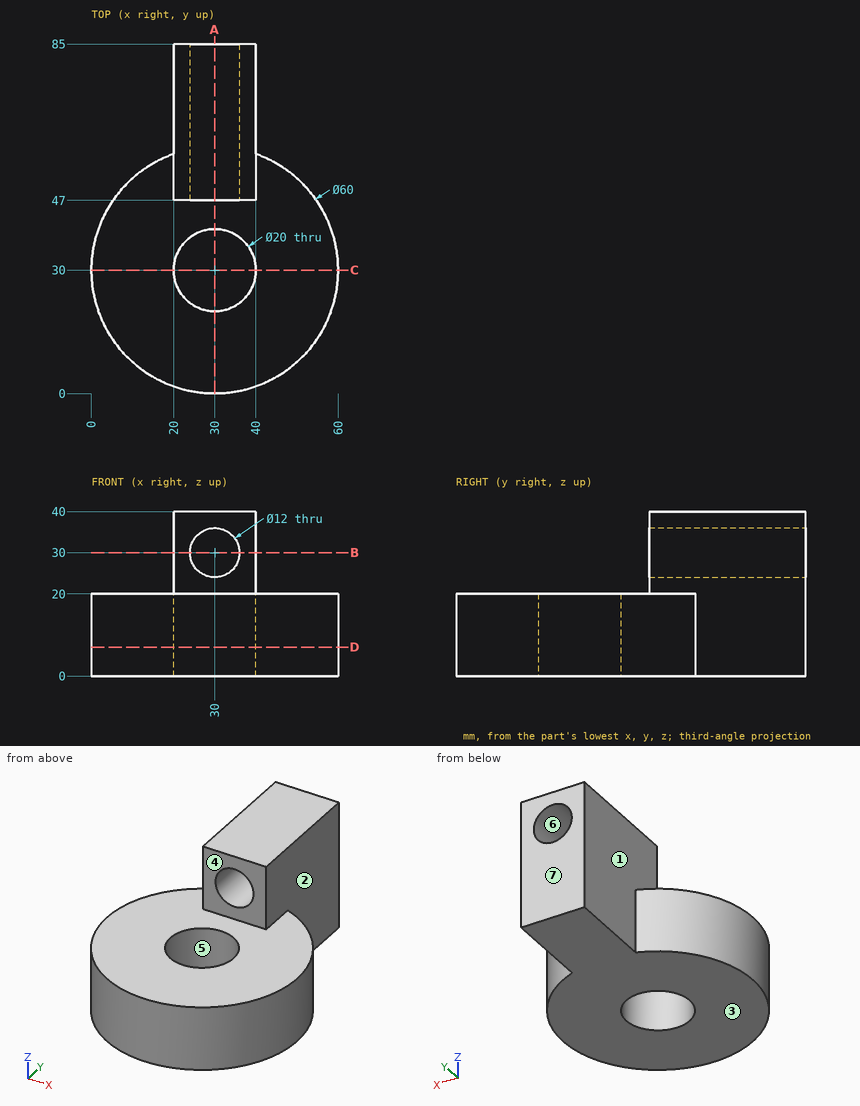
Geometry: see drawing. Coordinates: mm, zero at the bounding-box minimum. A direction names the side the tool comes from. Coordinates: 2 decimals unless noted, no trailing zeros. Order: outer loops, then holes, each group sorted by start corner. A loop starts at its lowest first (then second) coordinate and runs counter-clockwise, first axis right, second up. Notation, with made-up numbers: (40, -12) - (44, -12) arc R26 cw to (44, 27) - close; hole circle Ø5 at (-16, 72.25). An arc over 180 degrees is marked (long way). Write each question's results on one line, items separated by ' | '.
1) Section A-A, the plane x = 30. Return loops of the section in (y, z).
Results list:
outline: (0, 0) - (20, 0) - (20, 20) - (0, 20) - close; (40, 0) - (85, 0) - (85, 24) - (47, 24) - (47, 20) - (40, 20) - close; (47, 36) - (85, 36) - (85, 40) - (47, 40) - close
2) Section D-D, the plane z = 7. Return loops of the section in (x, y), plus the area to 3 significant figures.
Results list:
outline: (20, 58.28) arc R30 ccw (long way) to (40, 58.28) - (40, 85) - (20, 85) - close; hole circle Ø20 at (30, 30) | area: 3,020 mm^2
3) Set-up query: the marked faces 1, 2 and 3. Return all of +Z, -Z, +X, -X, +Y, -Y with unobstructed straight access to the full face (end or side cutting, diameter ignored); none if empty.
Results list:
face 1: +Z, -X, +Y | face 2: +Z, +X, +Y | face 3: -Z, +X, -X, +Y, -Y
4) Section B-B, the plane z = 30. Return loops of the section in (x, y), plus the area to 3 significant figures.
Results list:
outline: (20, 47) - (24, 47) - (24, 85) - (20, 85) - close; (36, 47) - (40, 47) - (40, 85) - (36, 85) - close | area: 304 mm^2
5) Pin query (flat end, axial travel): pin 1 (6 mm diameter, centred on x = 37.5, z = 14.5, fed in from -Y); pin 2 (7 mm diameter, centred on x = 30, z = 30, fed in from -Y) (3 decimals); pin 3 (4 mm diameter, centred on x = 46, z = 16.5, fed in from -Y); pin 4 (8 mm diameter, centred on x = 8.5, y = 36.5, fed in from +Z). Return the tip coordinate at first contact, or that it passes through.
Results list:
pin 1: y = 0.34 | pin 2: through | pin 3: y = 3.47 | pin 4: z = 20
6) Section C-C, the plane y = 30. Return loops of the section in (x, z), plus the area to 3 significant figures.
Results list:
outline: (0, 0) - (20, 0) - (20, 20) - (0, 20) - close; (40, 0) - (60, 0) - (60, 20) - (40, 20) - close | area: 800 mm^2
7) Pull-direction query (Y, two-part tool) for the marked faces 4, 5, 6 and 7; classes: pulls with the +Y half, pulls with the -Y half, needs draft (parallel to the pull), parting line crosses it, or undercut.
Results list:
face 4: pulls with the -Y half | face 5: undercut | face 6: needs draft | face 7: pulls with the +Y half
8) Line query: line 1 (Z direction, x = 30, y = 63); line 2 (X direction, y = 75, z = 30); line 3 (Y direction, x = 30, z = 5.75). Output: solid intervals per line, ascending. Write a range as from..to.
Results list:
line 1: 0..24, 36..40 | line 2: 20..24, 36..40 | line 3: 0..20, 40..85
